Autodesk Inventor part; units mm, degrees
ref_plane "YZ Plane" through (0, 0, 0) normal (1, 0, 0) x (0, 1, 0)
ref_plane "XZ Plane" through (0, 0, 0) normal (0, 1, 0) x (-1, 0, 0)
ref_plane "XY Plane" through (0, 0, 0) normal (0, 0, 1) x (1, 0, 0)
sketch "Sketch1" plane through (0, 0, 0) normal (0, 1, 0) x (-1, 0, 0)
  line L0 (0, 0) -> (-7, 0)
  line L1 (-7, 0) -> (-7, -7)
  line L2 (-7, -7) -> (0, -7)
  line L3 (0, -7) -> (0, 0)
  dimension "d0" = 7
  dimension "d1" = 7
extrude "Extrusion1" add sketch "Sketch1" along normal blind 46
sketch "Sketch2" plane through (0, 46, 0) normal (0, 1, 0) x (1, 0, 0)
  line L0 (0, 7) -> (0, 0)
  line L1 (0, 3.5) -> (7, 3.5)
  line L2 (7, 0) -> (7, 7)
  line L3 (7, 7) -> (0, 7)
  line L4 (3.5, 7) -> (3.5, 0)
  line L5 (0, 0) -> (7, 0)
  point P0 (3.5, 3.5)
hole "Hole1" at (3.5, 46, -3.5) direction (0, -1, 0) diameter 2.616 end through all
properties part number "Spacer" material "ABS Plastic"
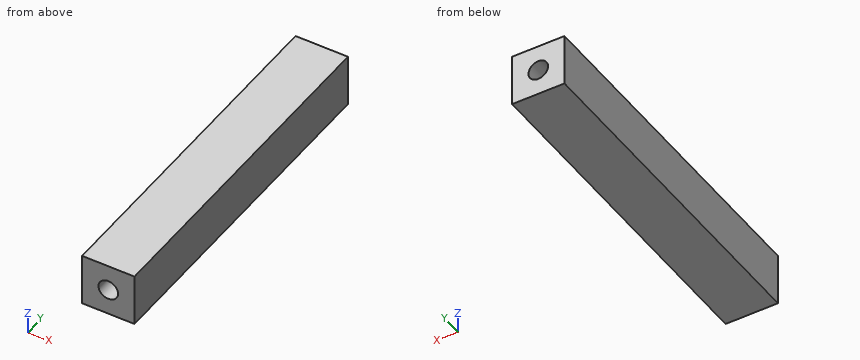
Geometry check sheet. Reference: the model listing, model coordinates, mm. Coordinates: 2 decimals unless noted, no trailing zeros. Order: outer loops, then holes, each group sorted by start corner. A loop starts at its lowest first (then second) coordinate and runs counter-clockwise, first axis right, second up. Notation, with made-up numbers: (34.5, 82) - (70.5, 82) arc R20 cw to (70.5, 116) - close; hole circle Ø8 at (6, 28). An arc over 180 degrees is marked (long way). Answer in a Markdown table with one row per item. Add a question column.
1) Material ranges on line 1 along Z through (x, y) = (3.5, 26); line 2 along X through (y, z) = (16, -3.5); line 3 along X through (y, z) = (21, -4), recorded low to high. Write a range as [from, to].
2) Cross-section at A-A, the plane x = 3.5. Record the cut outline in (y, z).
3) Gauge pin test, flat end, axial feed: P1, Ø2.5, axis at x = 3.5, z = -3.5, coming from the -Y side. Record the tip position at first contact, or that the pin passes through.
4) Cross-section at C-C, the plane y = 11. Record the cut outline in (x, z).
5) Cross-section at B-B, the plane z = -3.5. Record the cut outline in (x, y), then the cut area to 3 significant figures.
Check result:
| question | item | result |
|---|---|---|
| 1 | line 1 | z = [-7, -4.81], [-2.19, 0] |
| 1 | line 2 | x = [0, 2.19], [4.81, 7] |
| 1 | line 3 | x = [0, 2.29], [4.71, 7] |
| 2 | outline | (0, -7) - (46, -7) - (46, -4.81) - (0, -4.81) - close; (0, -2.19) - (46, -2.19) - (46, 0) - (0, 0) - close |
| 3 | P1 | passes through |
| 4 | outline | (0, -7) - (7, -7) - (7, 0) - (0, 0) - close; hole circle Ø2.62 at (3.5, -3.5) |
| 5 | outline | (0, 0) - (2.19, 0) - (2.19, 46) - (0, 46) - close; (4.81, 0) - (7, 0) - (7, 46) - (4.81, 46) - close |
| 5 | area | 202 mm² |
